CAD build for the part. Positions are in the model's coordinates, mm. A direction names the side the tool comes from. Give positions to 0.01 mm unless a question says otherwise; leave off trailing zeros. Order: outer loops, then holes, each group sorted by start corner. A loop starts at its lowest first (then second) coordinate and runs counter-clockwise, first axis right, second up.
Item 1: Two-plate mould, pull along X, no slides. Class faces 4 (the flat face through (15, 2, 5)), 5 (the cylindrical face through (13.25, 6.22, -1.27)), 6 (the flat face through (7, 2.5, 12)): released by +X, released by -X, zero draft, split by the parting line, or undercut.
Item 2: Which spindle directions (+Z, -Z, +X, -X, +Y, -Y) get a long thin tool onto all of the face, cutting with end or side? Do faces 1 (the cylindrical face through (8.25, 6.22, 11.16)), 2 (the flat face through (13, 6, 17.5)), 3 (the cylindrical face through (3.25, 6.22, -1.27)). Say none if no direction does.
Item 3: Band-saw the part on B-B on y = 6.25. Give the cut face in (x, z).
Item 4: Band-saw the part on C-C on x = 4.75. Give the cut face in (y, z).
Item 5: Band-saw the part on D-D on y = 4.25. Give the cut face in (x, z).
Item 6: Flat gauge pins, fed straight in: P1, Ø6, axis at x = 11.5, z = 7, coming from the -Y side; P2, Ø1.5, axis at x = 6, y = 5, coming from the -Z side; P3, Ø1.2, axis at x = 7, y = 6, coming from the +Z side; P4, Ø2, axis at x = 6, z = 7.5, coming from the +Y side. Where does each tip first touch, or does it go through?
Item 7: Band-saw the part on A-A on x = 7.5. Give the cut face in (y, z).
Item 8: Wall check: L1, parallel to X at y = 6, z = 12.5; L2, parallel to Y at x = 12.5, z = 7.5; L3, parallel to Z at x = 9.25, y = 8.5. Give the ranges that are in metal, low to high.
```python
from build123d import *

# Parameters (mm, degrees)
SKETCH_1_W           = 15
SKETCH_1_H           = 10
EXTRUDE_1_DEPTH      = 5
SKETCH_2_W           = 15
SKETCH_2_H           = 2.5
EXTRUDE_2_DEPTH      = 15
EXTRUDE_3_DEPTH      = 12.5
EXTRUDE_3_DEPTH_BACK = 7.5
SKETCH_3_R           = 0.75


with BuildPart() as part:
    # Sketch 1 → Extrude 1 (new body)
    with BuildSketch(Plane.XY):
        with Locations((7.5, 5)):
            Rectangle(SKETCH_1_W, SKETCH_1_H)
    extrude(amount=EXTRUDE_1_DEPTH)

    # Sketch 2 → Extrude 2 (add)
    with BuildSketch(Plane.XY.offset(5)):
        with Locations((7.5, 1.25)):
            Rectangle(SKETCH_2_W, SKETCH_2_H)
    extrude(amount=EXTRUDE_2_DEPTH)

    # Sketch 3 → Extrude 3 (add, two sides: drawn at the far end of the back side and taken through both)
    with BuildSketch(Plane.XY.offset(5).offset(-EXTRUDE_3_DEPTH_BACK)):
        with Locations(Location((7.5, 6.25, 0), (0, 0, 180))):
            Circle(SKETCH_3_R)
        with Locations(Location((12.5, 6.25, 0), (0, 0, 180))):
            Circle(SKETCH_3_R)
        with Locations(Location((2.5, 6.25, 0), (0, 0, 180))):
            Circle(SKETCH_3_R)
    extrude(amount=EXTRUDE_3_DEPTH + EXTRUDE_3_DEPTH_BACK)


solid = part.part
```
The answers:
1. face 4: released by +X
1. face 5: undercut
1. face 6: zero draft
2. face 1: +Z
2. face 2: +Z, +X, -X, +Y
2. face 3: -Z
3. outline: (0, 0) - (1.75, 0) - (1.75, -2.5) - (3.25, -2.5) - (3.25, 0) - (6.75, 0) - (6.75, -2.5) - (8.25, -2.5) - (8.25, 0) - (11.75, 0) - (11.75, -2.5) - (13.25, -2.5) - (13.25, 0) - (15, 0) - (15, 5) - (13.25, 5) - (13.25, 17.5) - (11.75, 17.5) - (11.75, 5) - (8.25, 5) - (8.25, 17.5) - (6.75, 17.5) - (6.75, 5) - (3.25, 5) - (3.25, 17.5) - (1.75, 17.5) - (1.75, 5) - (0, 5) - close
4. outline: (0, 0) - (10, 0) - (10, 5) - (2.5, 5) - (2.5, 20) - (0, 20) - close
5. outline: (0, 0) - (15, 0) - (15, 5) - (0, 5) - close
6. P1: stops at y = 0
6. P2: stops at z = 0
6. P3: stops at z = 17.5
6. P4: stops at y = 6.81
7. outline: (0, 0) - (5.5, 0) - (5.5, -2.5) - (7, -2.5) - (7, 0) - (10, 0) - (10, 5) - (7, 5) - (7, 17.5) - (5.5, 17.5) - (5.5, 5) - (2.5, 5) - (2.5, 20) - (0, 20) - close
8. L1: x = 1.79 to 3.21, 6.79 to 8.21, 11.79 to 13.21
8. L2: y = 0 to 2.5, 5.5 to 7
8. L3: z = 0 to 5
